Source: CAD feature listing. Evaluate the final solid. Frame: model axes, mm. Give positions to 0.01 mm unless a question says otherwise; leave off trailing zeros. Order: outer loops, then holes, each group sorted by start corner. A loop starts at its lowest first (then second) coordinate and runs counter-clockwise, first axis right, second up. Notation, with made-up numbers: M 1.25,30.25 L 38.25,30.25 A19 cw 38.25,34.25 Z; hole C 82.25,35.25 d2. An arc over 180 degrees is marked long. Return JSON: item names as keys, results as strings.
Autodesk Inventor part; units mm, degrees
ref_plane "YZ Plane" through (0, 0, 0) normal (1, 0, 0) x (0, 1, 0)
ref_plane "XZ Plane" through (0, 0, 0) normal (0, 1, 0) x (-1, 0, 0)
ref_plane "XY Plane" through (0, 0, 0) normal (0, 0, 1) x (1, 0, 0)
sketch "Sketch1" plane through (0, 0, 0) normal (0, 1, 0) x (-1, 0, 0)
  line L0 (15, 25) -> (-15, 25)
  line L1 (12.5, 0) -> (-12.5, 0)
  line L2 (6, -37.5) -> (-6, -37.5)
  line L3 (15, 25) -> (12.5, 0)
  line L4 (6, -37.5) -> (12.5, 0)
  line L5 (-15, 25) -> (-12.5, 0)
  line L6 (-12.5, 0) -> (-6, -37.5)
  line L7 (21, 0) -> (-21, 0)
  line L8 (0, -50) -> (0, 37.5)
  point P0 (0, 0)
  point P1 (0, 25)
  point P2 (0, 0)
  point P3 (0, -37.5)
  dimension "d0" = 30
  dimension "d1" = 25
  dimension "d2" = 12
  dimension "d3" = 25
  dimension "d4" = 37.5
extrude "Extrusion1" add sketch "Sketch1" along normal blind 14 contours L3 L1 L8 L0 | L8 L1 L5 L0
sketch "Sketch2" plane through (0, 0, 0) normal (0, 1, 0) x (-1, 0, 0)
  line L0 (6, -37.5) -> (-6, -37.5)
  line L1 (-12.5, 0) -> (12.5, 0)
  line L2 (12.5, 0) -> (15, 25)
  line L3 (12.5, 0) -> (6, -37.5)
  line L4 (-12.5, 0) -> (-6, -37.5)
  line L5 (12.5, 0) -> (-12.5, 0)
  point P0 (0, 0)
  point P1 (0, -37.5)
  point P2 (0, 0)
  dimension "d7" = 12
  dimension "d8" = 37.5
extrude "Extrusion2" add sketch "Sketch2" along normal blind 14
sketch "Sketch3" plane through (0, 0, 0) normal (1, 0, 0) x (0, 1, 0)
  line L0 (-2.8, 0) -> (16.8, 0)
  line L1 (0, -50) -> (0, 37.5)
  line L2 (0, -37.5) -> (14, -37.5)
  line L3 (14, -37.5) -> (14, 0)
  line L4 (0, -37.5) -> (0, 0)
  line L5 (14, 0) -> (14, 25)
  line L6 (0, 25) -> (14, 25)
  line L7 (0, 0) -> (14, 0)
  line L8 (0, -37.5) -> (2.25, -37.5)
  line L9 (2.25, -37.5) -> (14, 0)
  line L10 (14, 0) -> (14, -37.5)
  line L11 (2.25, -37.5) -> (14, -37.5)
  dimension "d11" = 2.25
extrude "Extrusion3" cut sketch "Sketch3" along normal through all both and the other way through all contours L3 L2 L9
sketch "Sketch4" plane through (0, 0, 0) normal (0, -1, 0) x (1, 0, 0)
  line L0 (12.5, 0) -> (6, -37.5)
  line L1 (12.0667, -2.5) -> (-12.0667, -2.5)
  line L2 (-6, -37.5) -> (-12.5, 0)
  line L3 (11.2, -7.5) -> (-11.2, -7.5)
  line L4 (-15, 25) -> (15, 25)
  line L5 (12.0667, -2.5) -> (11.2, -7.5)
  line L6 (-12.0667, -2.5) -> (-11.2, -7.5)
  point P0 (0, 0)
  dimension "d14" = 27.5
  dimension "d15" = 5
extrude "Extrusion4" cut sketch "Sketch4" against normal blind 5.5
properties part number "FP Front Hood"
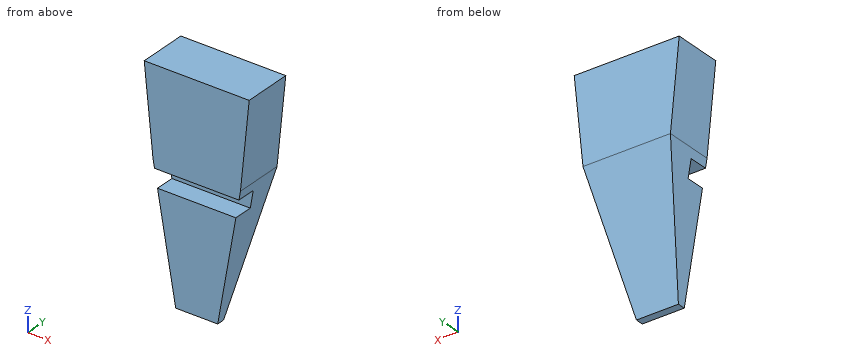
1. Section query B-B (x = -2.25). Return loops of the section in (y, z).
Evaluation:
{"outline": "M 0,-37.5 L 2.25,-37.5 L 14,0 L 14,25 L 0,25 L 0,-2.5 L 5.5,-2.5 L 5.5,-7.5 L 0,-7.5 Z"}
2. Section query A-A (y = 1). Return loops of the section in (x, z), then the cut area to 3 significant figures.
Evaluation:
{"outline": "M -15,25 L -12.5,0 L -12.07,-2.5 L 12.07,-2.5 L 12.5,0 L 15,25 Z; M -11.2,-7.5 L -6,-37.5 L 6,-37.5 L 11.2,-7.5 Z", "area": "1,260 mm^2"}
3. Section query C-C (z = 7). Return loops of the section in (x, y).
Evaluation:
{"outline": "M -13.2,0 L 13.2,0 L 13.2,14 L -13.2,14 Z"}
4. First-contact query: pin 1 (3 mm diameter, centred on y = 9, z = 10.5, fed in from +X); pin 2 (3 mm diameter, centred on y = 1.5, z = -7.5, fed in from -X); pin 3 (8 mm diameter, centred on y = 12, z = 2.5, fed in from -X); pin 4 (2 mm diameter, centred on x = -10, z = -22, fed in from +Y). Flat tips, straight axial feed; report the tip coordinate or a pass-through.
Evaluation:
{"pin 1": "stops at x = 13.7", "pin 2": "stops at x = -11.2", "pin 3": "stops at x = -13.15", "pin 4": "passes through"}
5. Section query D-D (y = 6.25). Return loops of the section in (x, z), then the cut area to 3 significant figures.
Evaluation:
{"outline": "M -15,25 L -12.5,0 L -8.21,-24.73 L 8.21,-24.73 L 12.5,0 L 15,25 Z", "area": "1,200 mm^2"}
6. Ray query, probe 1 along X at (y, z) = (10, 2); probe 2 along Z at (x, y) = (11.5, 3); probe 3 along X at (y, z) = (2.25, -2). Return the intervals inside material, ascending.
Evaluation:
{"probe 1": "x = -12.7 to 12.7", "probe 2": "z = -2.5 to 25", "probe 3": "x = -12.15 to 12.15"}
